from build123d import *

# Parameters (mm, degrees)
CHAMFER1_SIZE      = 1.25
FILLET1_R          = 0.4
CUT_EXTRUDE1_DEPTH = 4.5


with BuildPart() as part:
    # Sketch1 → Revolve1 (revolve)
    with BuildSketch(Plane.XY, mode=Mode.PRIVATE) as revolve1_sk:
        Polygon((0, 0), (0, 24), (-6.5, 24), (-6.5, 16), (-4, 16), (-4, 0), align=None)
    revolve(revolve1_sk.sketch.rotate(Axis((0, 0, 0), (0, 1, 0)), 270), axis=Axis((0, 0, 0), (0, 1, 0)))

    # Chamfer1
    chamfer1_edges = [part.edges().sort_by_distance(p)[0] for p in [
        (0, 0, 4),
    ]]
    chamfer(chamfer1_edges, length=CHAMFER1_SIZE)

    # Fillet1
    fillet1_edges = [part.edges().sort_by_distance(p)[0] for p in [
        (0, 24, 6.5),
    ]]
    fillet(fillet1_edges, radius=FILLET1_R)

    # Sketch2 → Cut-Extrude1 (cut)
    with BuildSketch(Plane(origin=(0, 24, 0), x_dir=(1, 0, 0), z_dir=(0, 1, 0))):
        Polygon((-4, 0), (-2, -3.464101615), (2, -3.464101615), (4, 0), (2, 3.464101615), (-2, 3.464101615), align=None)
    extrude(amount=-CUT_EXTRUDE1_DEPTH, mode=Mode.SUBTRACT)

    # Sketch3 → Cut-Revolve1 (revolve, cut)
    with BuildSketch(Plane.XY, mode=Mode.PRIVATE) as cut_revolve1_sk:
        Polygon((4, 19.5), (0, 18.5), (0, 19.5), align=None)
    revolve(cut_revolve1_sk.sketch.rotate(Axis((0, 18.5, 0), (0, 1, 0)), 270), axis=Axis((0, 18.5, 0), (0, 1, 0)), mode=Mode.SUBTRACT)


solid = part.part
Can you work these out from the model? Positions are in its coordinate system, mm. A direction names the side the tool comes from. Round coordinates to 2 decimals unless told otherwise and drop trailing zeros. Write each loop counter-clockwise with the first axis right and the second up, starting at its lowest first coordinate (ties: lowest second). Pieces come first, ordered by that corner, then holes. Notation, with made-up numbers: (26.25, 64) - (78.25, 64) arc R27 ccw to (78.25, 92) - close; hole circle Ø6 at (63, 81). An arc over 180 degrees is marked (long way). Write each question's results on one line, items separated by ' | '. Start each with the question number.
1) Please list where these lines run through material, in increasing order: line 1 (Y direction, x = 1.25, z = 4); line 2 (X direction, y = 19.75, z = -2.25); line 3 (X direction, y = 20, z = -0.75).
2) For pin 1 Ø1 at (x, z) = (-3, 2.5) entering from -Y; pin 2 Ø0.6 at (x, z) = (3.5, 2) entering from -Y; pin 3 Ø0.6 at (x, z) = (-3, -2) entering from -Y, each with a flat end and sliding along its axis, tell me the tip position at first contact or that it passes through.
3) We'd pull the mould along X, two halves only. Please class faces 4 (the cylindrical face through (3.955, 19.747, 5.158)), 5 (the flat face through (0, 0, 0)), 6 (the flat face through (0, 22, 3.464)): released by +X, released by -X, zero draft, split by the parting line, or undercut.
4) Suppose I cut it at A-A (y = 16.5). List the corners of the cut face in (x, z) for me.
5) Which directions (+Z, -Z, +X, -X, +Y, -Y) give clear straight access to the entire face, cutting with the end or side of a thin tool? Please do faces 1 (the cylindrical face through (3.905, 8.522, 0.867)), 2 (the flat face through (3, 24, 3)), 3 (the flat face through (-3.014, 21.782, 1.708)).
6) Suppose I cut it at B-B (y = 14). List the corners of the cut face in (x, z) for me.
Here are the results:
1) line 1: y = 16 to 24 | line 2: x = -6.1 to -2.7, 2.7 to 6.1 | line 3: x = -6.46 to -3.57, 3.57 to 6.46
2) pin 1: stops at y = 0.66 | pin 2: stops at y = 0.98 | pin 3: stops at y = 0.56
3) face 4: split by the parting line | face 5: zero draft | face 6: undercut
4) outline: circle Ø13 at (0, 0)
5) face 1: -Y | face 2: +Z, -Z, +X, -X, +Y | face 3: +Y
6) outline: circle Ø8 at (0, 0)
